Read the model definition and answer for the solid it produces. Units are mm, in the model's axes. A direction names the side the tool comes from. Coordinates: 2 decimals unless noted, no trailing zeros. Order: outer loops, then holes, each group sorted by start corner. A loop starts at its lowest first (then second) coordinate and runs counter-clockwise, first axis right, second up. Notation, with made-up numbers: (65, 87.5) -> (79, 87.5) arc R33 cw to (79, 116.5) -> close; hole circle Ø6 at (-16.75, -9.5). An arc over 180 degrees is marked (long way). Return JSON: item names as keys, results as strings. Group by question number.
```python
from build123d import *

# Parameters (mm, degrees)
BOSS_EXTRUDE1_DEPTH = 116.3
CUT_EXTRUDE1_DEPTH  = 112.7
FILLET1_R           = 2


with BuildPart() as part:
    # Sketch1 → Boss-Extrude1 (new body)
    with BuildSketch(Plane.XY):
        with BuildLine():
            Line((0, 0), (59.04, 0))
            Line((59.04, 0), (59.04, 4.82))
            ThreePointArc((59.04, 4.82), (57.136194078, 9.416194078), (52.54, 11.32))
            Line((52.54, 11.32), (6.5, 11.32))
            ThreePointArc((6.5, 11.32), (1.903805922, 9.416194078), (0, 4.82))
            Line((0, 4.82), (0, 0))
        make_face()
    extrude(amount=BOSS_EXTRUDE1_DEPTH)

    # Sketch2 → Cut-Extrude1 (cut)
    with BuildSketch(Plane.XY.offset(116.3)):
        with BuildLine():
            Line((1.8, 4.82), (1.8, 2.05))
            Line((1.8, 2.05), (1.8, 0.78))
            Line((1.8, 0.78), (1.8, 0))
            Line((1.8, 0), (57.24, 0))
            Line((57.24, 0), (57.24, 0.78))
            Line((57.24, 0.78), (57.24, 2.05))
            Line((57.24, 2.05), (57.24, 4.82))
            ThreePointArc((57.24, 4.82), (55.863401872, 8.143401872), (52.54, 9.52))
            Line((52.54, 9.52), (6.5, 9.52))
            ThreePointArc((6.5, 9.52), (3.176598128, 8.143401872), (1.8, 4.82))
        make_face()
        Polygon((57.24, 2.05), (57.24, 0.78), (57.895, 2.05), align=None)
        Polygon((1.8, 0.78), (1.8, 2.05), (1.145, 2.05), align=None)
    extrude(amount=-CUT_EXTRUDE1_DEPTH, mode=Mode.SUBTRACT)

    # Fillet1
    fillet1_edges = [part.edges().sort_by_distance(p)[0] for p in [
        (1.903805922, 9.416194078, 0),
        (29.52, 11.32, 0),
        (57.136194078, 9.416194078, 0),
        (59.04, 2.41, 0),
        (0, 2.41, 0),
    ]]
    fillet(fillet1_edges, radius=FILLET1_R)


solid = part.part
```
1. Find section A-A on z = 7.5. Determine the outline of the cut face in (x, y) (3 decimals), and give its area (3 significant figures).
2. Given pin 1 (4 mm diameter, centred on x = 29.5, y = 9.5, fed in from -Z); pin 2 (2 mm diameter, centred on x = 19.5, y = 3, fed in from +Z); pin 3 (6 mm diameter, centred on x = 35, z = 66.5, fed in from -Y), each flat-ended and moving along its own axis, determine where each tip first touches the part or whether it passes through.
3. Which of the six approach directions +Z, -Z, +X, -X, +Y, -Y give full straight-line access (tool end or side, diameter ignored) to faces 4 (the face through (30, 9.52, 61)), 5 (the face through (30, 11.32, 58))?
4. Find section B-B on x = 50. Determine the outline of the cut face in (y, z).
5. For a pull along X with two mould halves and no side action, classify faces 1 (the face through (0.6, 2.38, 0.57)), 2 (the face through (3.213, 8.18, 60.739)), 3 (the face through (29.2, 10.72, 0.57)) as released by +X, released by -X, zero draft, split by the parting line, or undercut.
6. Straight lines are drawn through the part: L1, parallel to Z at x = 34, y = 7.75; L2, parallel to Y at x = 35.5, z = 22; L3, parallel to X at y = 9, z = 15. For each, find the intervals that lie inside material, in ascending order.
Result:
{
 "1": {"outline": "(0, 0) -> (1.8, 0) -> (1.8, 0.78) -> (1.145, 2.05) -> (1.8, 2.05) -> (1.8, 4.82) arc R4.7 cw to (6.5, 9.52) -> (52.54, 9.52) arc R4.7 cw to (57.24, 4.82) -> (57.24, 2.05) -> (57.895, 2.05) -> (57.24, 0.78) -> (57.24, 0) -> (59.04, 0) -> (59.04, 4.82) arc R6.5 ccw to (52.54, 11.32) -> (6.5, 11.32) arc R6.5 ccw to (0, 4.82) -> close", "area": "131 mm^2"},
 "2": {"pin 1": "z = 0", "pin 2": "z = 3.6", "pin 3": "y = 9.52"},
 "3": {"face 4": "+Z, -Y", "face 5": "+Z, -Z, +X, -X, +Y"},
 "4": {"outline": "(0, 0) -> (9.32, 0) arc R2 ccw to (11.32, 2) -> (11.32, 116.3) -> (9.52, 116.3) -> (9.52, 3.6) -> (0, 3.6) -> close"},
 "5": {"face 1": "released by -X", "face 2": "undercut", "face 3": "zero draft"},
 "6": {"L1": "0 to 3.6", "L2": "9.52 to 11.32", "L3": "1.52 to 4.35, 54.69 to 57.52"}
}
